```python
from build123d import *

# Parameters (mm, degrees)
F0_W     = 100.5
F0_H     = 33.5
F1_DEPTH = 5
F0_W_2   = 110.5
F0_H_2   = 43.5
F2_DEPTH = 37
F3_R     = 5


with BuildPart() as f1:
    # F0 (on Top) → F1 (new body)
    with BuildSketch(Plane.XY):
        Rectangle(F0_W, F0_H)
    extrude(amount=F1_DEPTH)

    # F0 (on Top) → F2 (join)
    with BuildSketch(Plane.XY):
        Rectangle(F0_W_2, F0_H_2)
        Rectangle(F0_W, F0_H, mode=Mode.SUBTRACT)
    extrude(amount=F2_DEPTH)

    # F3
    f3_edges = [f1.edges().sort_by_distance(p)[0] for p in [
        (-55.25, 0, 0),
        (0, 21.75, 0),
        (55.25, 0, 0),
        (0, -21.75, 0),
    ]]
    fillet(f3_edges, radius=F3_R)


solid = f1.part
```
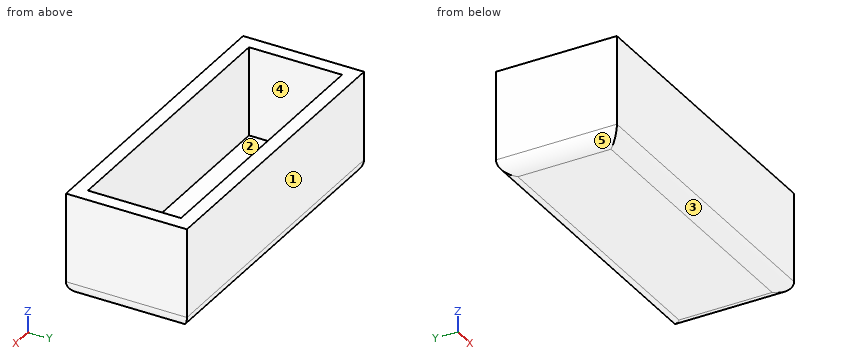
Here's how the part is built. I have some questions about the finished solid (model axes, mm). Face numbers are marked on the shaded views. A direction names the side the tool comes from. Coordinates: 2 decimals unless noted, no trailing zeros. Order: outer loops, then holes, each group sorted by start corner. A loop starts at its lowest first (then second) coordinate and runs counter-clockwise, first axis right, second up.
Item 1: If we section it at A-A, the plane z = 21: List the corners of the cut face in (x, y) for me, then the cut area to 3 significant figures.
Response values:
outline: (-55.25, -21.75) - (55.25, -21.75) - (55.25, 21.75) - (-55.25, 21.75) - close; hole (-50.25, -16.75) - (50.25, -16.75) - (50.25, 16.75) - (-50.25, 16.75) - close
area: 1,440 mm2
Item 2: If we section it at B-B, the plane y = 5.5: List the corners of the cut face in (x, z) for me.
Response values:
outline: (-55.25, 5) arc R5 ccw to (-50.25, 0) - (50.25, 0) arc R5 ccw to (55.25, 5) - (55.25, 37) - (50.25, 37) - (50.25, 5) - (-50.25, 5) - (-50.25, 37) - (-55.25, 37) - close
Item 3: If we section it at C-C, the plane x = -14: List the corners of the cut face in (y, z) for me, then the cut area to 3 significant figures.
Response values:
outline: (-21.75, 5) arc R5 ccw to (-16.75, 0) - (16.75, 0) arc R5 ccw to (21.75, 5) - (21.75, 37) - (16.75, 37) - (16.75, 5) - (-16.75, 5) - (-16.75, 37) - (-21.75, 37) - close
area: 527 mm2
Item 4: Which directions (+Z, -Z, +X, -X, +Y, -Y) give clear straight access to the entire face, cutting with the end or side of a thin tool? Please do the marked faces 1 and 2.
Response values:
face 1: +Z, -Z, +X, -X, +Y
face 2: +Z
Item 5: I need wall thicknesses on probe 1 along Y at (x, z) = (-16, 26); probe 2 along X at (y, z) = (9.5, 29.5); probe 3 along Z at (x, y) = (-41.5, 12). Which ranges of each line are inside material? Lowest first, please.
Response values:
probe 1: y = -21.75 to -16.75, 16.75 to 21.75
probe 2: x = -55.25 to -50.25, 50.25 to 55.25
probe 3: z = 0 to 5
Item 6: I'm going to push a flat-ended pin straight in: pin 1 Ø4 at (x, y) = (22, -6.5) entering from +Z. Where does the tip first touch, or does it pass through?
Response values:
pin 1: stops at z = 5
Item 7: Thinking about a two-plate mould opening in Y: for the marked faces 3, 4 and 5, which applies, pulls with the +Y half, pulls with the -Y half, needs draft (parallel to the pull), parting line crosses it, or undercut?
Response values:
face 3: pulls with the -Y half
face 4: undercut
face 5: needs draft
Item 8: If we section it at D-D, the plane y = 19: List the corners of the cut face in (x, z) for me.
Response values:
outline: (-55.25, 5) arc R5 ccw to (-52.5, 0.53) - (52.5, 0.53) arc R5 ccw to (55.25, 5) - (55.25, 37) - (-55.25, 37) - close
